Check sheet for the modelled part. Datum: model origin and axes. Units: mm. A direction names the side the tool comes from. Round coordinates to 2 decimals unless told otherwise and drop trailing zeros. Write each loop counter-clockwise with the first axis right and the second up, starting at its lowest first coordinate (ties: lowest second). Pieces come first, ordered by that corner, then holes.
Autodesk Inventor part; units mm, degrees
ref_plane "YZ Plane" through (0, 0, 0) normal (1, 0, 0) x (0, 1, 0)
ref_plane "XZ Plane" through (0, 0, 0) normal (0, 1, 0) x (-1, 0, 0)
ref_plane "XY Plane" through (0, 0, 0) normal (0, 0, 1) x (1, 0, 0)
sketch "Sketch1" plane through (0, 0, 0) normal (0, 1, 0) x (-1, 0, 0)
  circle A0 centre (0, 0) radius 4.2
  line L0 (11.4529, -8.6044) -> (5.0517, -7.4757) construction
  line L1 (5.0517, -7.4757) -> (-4.499, -61.6402) construction
  line L2 (-4.499, -61.6402) -> (1.9023, -62.7689) construction
  line L3 (1.9023, -62.7689) -> (11.4529, -8.6044) construction
  line L4 (-3.9483, 8.1127) -> (-1.7252, 14.2207) construction
  line L5 (-1.7252, 14.2207) -> (-53.4083, 33.0318) construction
  line L6 (-53.4083, 33.0318) -> (-55.6314, 26.9238) construction
  line L7 (-55.6314, 26.9238) -> (-3.9483, 8.1127) construction
  arc A1 (11.4529, -8.6044) -> (-1.7252, 14.2207) centre (-10.3924, -6.0001) ccw
  line L8 (-3.9483, 8.1127) -> (-55.6314, 8.1127) construction
  line L9 (5.0517, -7.4757) -> (-3.9483, 8.1127) construction
  line L10 (0.5517, 0.3185) -> (-10.3924, -6.0001) construction
  line L11 (2.1781, -23.7726) -> (-19.4986, 13.7726)
  line L12 (11.4529, -8.6044) -> (5.0517, -7.4757)
  line L13 (5.0517, -7.4757) -> (2.1781, -23.7726)
  line L14 (-19.4986, 13.7726) -> (-3.9483, 8.1127)
  line L15 (-3.9483, 8.1127) -> (-1.7252, 14.2207)
  dimension "d0" = 8.4
  dimension "d2" = 6.5
  dimension "d3" = 55
  dimension "d4" = 100
  dimension "d5" = 22
  dimension "d6" = 18
  dimension "d7" = 20
  dimension "d8" = 0.637
  dimension "d9" = 10
extrude "Extrusion1" add sketch "Sketch1" along normal blind 95
properties part number "filament_guide_spool" material "ABS Plastic"
1. Scan lines: line 1 along Z through (x, y) = (-1, 52); line 2 along Z through (x, y) = (1.5, 42.5); line 3 along X through (y, z) = (21.5, -15.5). Record each from-to range of solid material in increasing order.
2. Sectioned sample at B-B, the plane x = 0. Enter the section's corners in (y, z), plus the area to 3 significant figures.
3. Sectioned sample at D-D, the plane x = -7.5. Enter the section's corners in (y, z), plus the area to 3 significant figures.
4. Sectioned sample at C-C, the plane z = 0. Enter the section's corners in (x, y), plus the area to 3 significant figures.
5. Release check for a two-part mould opening along Z. For faces 4 (the cylindrical face through (-4.006, 46.835, -1.262)), 5 (the flat face through (1, 0, -5)), 6 (the flat face through (8.51, 46.84, -5.26)) record: released by +Z, released by -Z, zero draft, split by the parting line, or undercut.
6. Go/stop test with flat-tipped pins: pin 1 (3 mm diameter, centred on x = 7, y = 44.5, fed in from -Z); pin 2 (1 mm diameter, centred on y = 50, z = 7, fed in from +X); pin 3 (6 mm diameter, centred on y = 26.5, z = -13, fed in from +X). Record where each tip stops, or that it passes through.
7. Sectioned sample at A-A, the plane y = 18. Enter the section's corners in (x, z).
8. Set-up check for faces 1 (the flat face through (1, 95, -5)), 2 (the flat face through (2.852, 46.835, 11.124)), 3 (the flat face through (-8.3, 46.84, -8.05)): record each of +Z, -Z, +X, -X, +Y, -Y from which the full face is reachable in a straight line by a thin tool's end or side.
Computed values:
1. line 1: z = -21.73 to -4.08, 4.08 to 12.82
1. line 2: z = -17.4 to -3.92, 3.92 to 14.12
1. line 3: x = -3.64 to 2.6
2. outline: (0, -20) - (95, -20) - (95, -4.2) - (0, -4.2) - close; (0, 4.2) - (95, 4.2) - (95, 13.39) - (0, 13.39) - close
2. area: 2,370 mm2
3. outline: (0, -7.91) - (95, -7.91) - (95, 6.8) - (0, 6.8) - close
3. area: 1,400 mm2
4. outline: (-10.77, 0) - (-4.2, 0) - (-4.2, 95) - (-10.77, 95) - close; (4.2, 0) - (11.55, 0) - (11.55, 95) - (4.2, 95) - close
4. area: 1,320 mm2
5. face 4: undercut
5. face 5: zero draft
5. face 6: released by -Z
6. pin 1: stops at z = -10.47
6. pin 2: stops at x = 15.88
6. pin 3: stops at x = 5.77
7. outline: (-11.45, -8.6) - (-5.05, -7.48) - (-2.18, -23.77) - (19.5, 13.77) - (3.95, 8.11) - (1.73, 14.22) arc R22 ccw to start; hole circle Ø8.4 at (0, 0)
8. face 1: +Z, -Z, +X, -X, +Y
8. face 2: +Z, +Y, -Y
8. face 3: -Z, +Y, -Y
